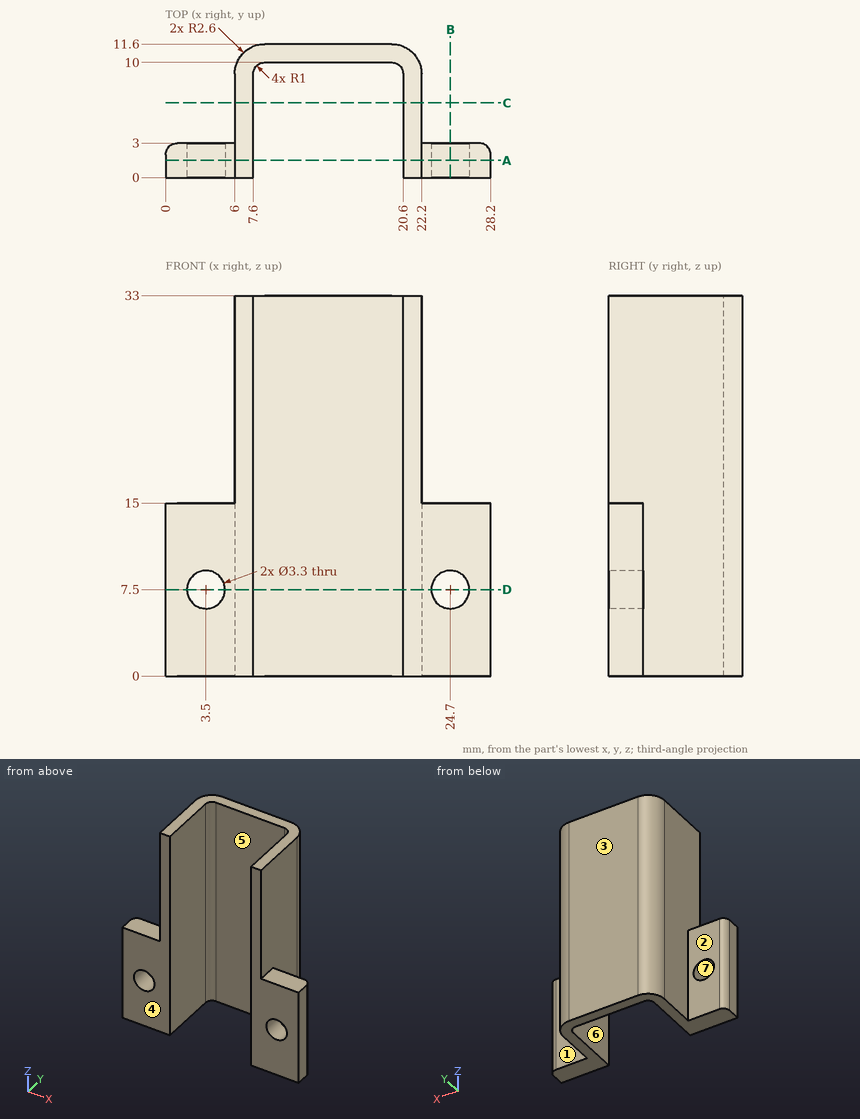
Could you check a few things on this drawing? It's one solid part, dimensions in mm from its lowest x, y, z. A direction names the side the tool comes from. Round coordinates to 2 decimals unless told otherwise and drop trailing zeros. Write each loop counter-clockwise with the first axis right and the second up, starting at its lowest first coordinate (ties: lowest second). Pieces come first, ordered by that corner, then holes.
Q1. Please list where these lines run through material, in increasing order: probe 1 along Z at (x, y) = (3.5, 1.6); probe 2 along X at (y, z) = (4, 12); probe 3 along Y at (x, z) = (13.5, 22.5).
Q2. Will these pins go through, and if not, where does the flat tip stop? P1, Ø1.5, axis at x = 3, y = 1, coming from the +Z side; P2, Ø1.5, axis at x = 23.5, z = 9.5, coming from the +Y side; P3, Ø2, axis at x = 6, z = 15.5, coming from the +Y side.
Q3. If we section it at A-A on y = 1.5: Write out the boundary of the cut face in (x, z), plus the area to 3 significant figures.
Q4. If we section it at B-B on x = 24.7: Write out the boundary of the cut face in (y, z).
Q5. If we section it at C-C on y = 6.5: Write out the boundary of the cut face in (x, z).
Q6. If we mould it in two halves opening along Z, with no side actions, what happens to the marked faces 6 and 7? For each: +Z half, -Z half, draft (parallel to the pull), parting line (faces both ways), or undercut.
Q7. Which directions (+Z, -Z, +X, -X, +Y, -Y) give clear straight access to the entire face, cutting with the end or side of a thin tool? Please do the marked faces 1, 2, 3, 4 and 5.
Q8. If we section it at D-D on z = 7.5: Write out the boundary of the cut face in (x, y).
Answer below:
1. probe 1: z = 0 to 5.85, 9.15 to 15
1. probe 2: x = 6 to 7.6, 20.6 to 22.2
1. probe 3: y = 10 to 11.6
2. P1: stops at z = 15
2. P2: stops at y = 3
2. P3: stops at y = 11.05
3. outline: (0, 0) - (7.6, 0) - (7.6, 33) - (6, 33) - (6, 15) - (0, 15) - close; (20.6, 0) - (28.2, 0) - (28.2, 15) - (22.2, 15) - (22.2, 33) - (20.6, 33) - close; hole circle Ø3.3 at (3.5, 7.5); hole circle Ø3.3 at (24.7, 7.5)
3. area: 268 mm2
4. outline: (0, 0) - (3, 0) - (3, 5.85) - (0, 5.85) - close; (0, 9.15) - (3, 9.15) - (3, 15) - (0, 15) - close
5. outline: (6, 0) - (7.6, 0) - (7.6, 33) - (6, 33) - close; (20.6, 0) - (22.2, 0) - (22.2, 33) - (20.6, 33) - close
6. face 6: draft
6. face 7: undercut
7. face 1: +Z, -Z, +X, +Y
7. face 2: +Z, -Z, -X, +Y
7. face 3: +Z, -Z, +X, -X, +Y
7. face 4: +Z, -Z, +X, -X, -Y
7. face 5: +Z, -Z, -Y
8. outline: (0, 0) - (1.85, 0) - (1.85, 3) - (1, 3) arc R1 ccw to (0, 2) - close; (5.15, 0) - (7.6, 0) - (7.6, 9) arc R1 cw to (8.6, 10) - (19.6, 10) arc R1 cw to (20.6, 9) - (20.6, 0) - (23.05, 0) - (23.05, 3) - (22.2, 3) - (22.2, 9) arc R2.6 ccw to (19.6, 11.6) - (8.6, 11.6) arc R2.6 ccw to (6, 9) - (6, 3) - (5.15, 3) - close; (26.35, 0) - (28.2, 0) - (28.2, 2) arc R1 ccw to (27.2, 3) - (26.35, 3) - close
